For this review, take the finished solid that the model builds, in its own axes (mm). Face numbers are marked on the shaded views. A direction names the side the tool comes from. Round coordinates to 2 decimals unless told otherwise and drop trailing zeros. Order: outer loops, then holes, each group sorted by start corner. A loop starts at its lowest first (then second) coordinate and runs counter-clockwise, first axis right, second up. Notation, with made-up numbers: M -32,89.25 L -2,89.25 A15 ccw -2,96.25 Z; hole C 8.5,27 d1. An arc over 180 degrees is marked long. Answer in a Markdown table with one row per item. Add a question column.
```python
from build123d import *

# Parameters (mm, degrees)
SKETCH003_R  = 1
PAD001_DEPTH = 25.5


with BuildPart() as part:
    # Sketch003 → Pad001 (new body)
    with BuildSketch(Plane(origin=(0, 0, 0), x_dir=(0, 1, 0), z_dir=(0, 0, 1))):
        Polygon((20.2, 20.2), (20.2, -20.2), (-20.2, -20.2), (-20.2, -10.1), (-29.4, -10.1), (-29.4, 10.1), (-20.2, 10.1), (-20.2, 20.2), (-10.1, 20.2), (-10.1, 29.4), (10.1, 29.4), (10.1, 20.2), align=None)
        with Locations((-16.25, 16.25)):
            Circle(SKETCH003_R, mode=Mode.SUBTRACT)
        with Locations((16.25, 16.25)):
            Circle(SKETCH003_R, mode=Mode.SUBTRACT)
        with Locations((16.25, -16.25)):
            Circle(SKETCH003_R, mode=Mode.SUBTRACT)
        with Locations((-16.25, -16.25)):
            Circle(SKETCH003_R, mode=Mode.SUBTRACT)
    extrude(amount=PAD001_DEPTH)

    # Sketch004 → Revolution (revolve)
    with BuildSketch(Plane.XZ):
        Polygon((0, 84), (12.31, 84), (17.5, 75.9), (17.5, 59.3), (5.833333, 44.5), (5.833333, 12.75), (0, 12.75), align=None)
    revolve(axis=Axis((0, 0, 0), (0, 0, 1)))


solid = part.part
```
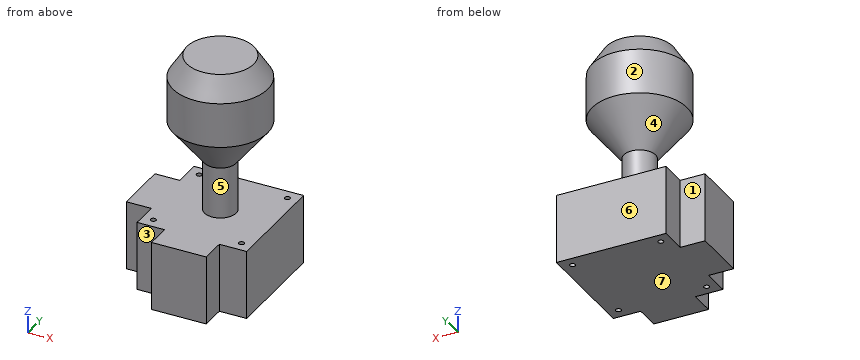
1. To check wall thickness, follow probe 1 along X at (y, z) = (-16.25, 15.5); probe 2 along Z at (x, y) = (-8.5, 2). State the ranges of each line that lie inside material, in increasing order. Write a range as [from, to].
2. Consider section D-D on z = 51. Write out the cut boundary in (x, y).
3. Consider section A-A on z = 13.5. Write out the cut boundary in (x, y).
4. For the marked faces 1, 2, 3 and 4, list the 3-axis set-ups (+Z, -Z, +X, -X, +Y, -Y) from which the entire face can be reached by the end or side of a thin tool; tool diameter is ignored.
5. Consider section B-B on x = 0. Write out the cut boundary in (y, z), plus the area to 3 significant figures.
6. Consider section C-C on y = -16.25. State how many separate pieces and enclosed holes the cut face has, plus the area to 3 significant figures.
7. Clearance check with flat-ended pins moving along their axes: pin 1 Ø11 at (y, z) = (-17, 14.5) entering from -X; pin 2 Ø6 at (x, z) = (-16, 65) entering from +Y; pin 3 Ø6 at (x, y) = (-9.5, -24) entering from +Z; pin 4 Ø4 at (x, y) = (-2, -2) entering from -Z. State where each tip first meets the part, or that it passes through.
8. The part is to be moulded in two halves that separate along Z. For the marked faces 5, 6 and 7, say which applies: pulls with the +Z half, pulls with the -Z half, needs draft (parallel to the pull), parting line crosses it, or undercut.
Solved:
| question | item | result |
|---|---|---|
| 1 | probe 1 | x = [-20.2, -17.25], [-15.25, 15.25], [17.25, 20.2] |
| 1 | probe 2 | z = [0, 25.5], [48.18, 84] |
| 2 | outline | C 0,0 d21.91 |
| 3 | outline | M -29.4,-10.1 L -20.2,-10.1 L -20.2,-20.2 L -10.1,-20.2 L -10.1,-29.4 L 10.1,-29.4 L 10.1,-20.2 L 20.2,-20.2 L 20.2,20.2 L -20.2,20.2 L -20.2,10.1 L -29.4,10.1 Z; hole C -16.25,-16.25 d2; hole C -16.25,16.25 d2; hole C 16.25,-16.25 d2; hole C 16.25,16.25 d2 |
| 4 | face 1 | +Z, -Z, -X, +Y |
| 4 | face 2 | +Z |
| 4 | face 3 | +Z, -Z, -X, -Y |
| 4 | face 4 | none |
| 5 | outline | M -29.4,0 L 20.2,0 L 20.2,25.5 L 5.83,25.5 L 5.83,44.5 L 17.5,59.3 L 17.5,75.9 L 12.31,84 L -12.31,84 L -17.5,75.9 L -17.5,59.3 L -5.83,44.5 L -5.83,25.5 L -29.4,25.5 Z |
| 5 | area | 2,650 mm^2 |
| 6 | separate pieces | 4 |
| 6 | enclosed holes | 0 |
| 6 | area | 1,170 mm^2 |
| 7 | pin 1 | stops at x = -20.2 |
| 7 | pin 2 | stops at y = 11.72 |
| 7 | pin 3 | stops at z = 25.5 |
| 7 | pin 4 | stops at z = 0 |
| 8 | face 5 | undercut |
| 8 | face 6 | needs draft |
| 8 | face 7 | pulls with the -Z half |
